Build history of the part. All positions in model axes, mm. A direction names the side the tool comes from. Round coordinates to 2 decimals unless told otherwise and drop trailing zeros. Write each loop counter-clockwise with the first axis right and the second up, starting at its lowest first coordinate (ties: lowest second). Pieces come first, ordered by that corner, then holes. Notation, with made-up numbers: (22, -37) - (46, -37) arc R22 cw to (46, -4) - close; hole circle Ø8 at (-11, -29.5). An arc over 180 degrees is marked (long way). Write each question's results on one line, items separated by ' | '.
from build123d import *

# Parameters (mm, degrees)
SKETCH1_W            = 186
SKETCH1_H            = 166
BOSS_EXTRUDE6_DEPTH  = 3
SKETCH9_W            = 183
SKETCH9_H            = 3
BOSS_EXTRUDE7_DEPTH  = 105
SKETCH8_W            = 3
SKETCH8_H            = 163
BOSS_EXTRUDE8_DEPTH  = 105
SKETCH7_W            = 186
SKETCH7_H            = 3
BOSS_EXTRUDE9_DEPTH  = 105
SKETCH11_W           = 3
SKETCH11_H           = 160
BOSS_EXTRUDE10_DEPTH = 105
SKETCH12_W           = 180
SKETCH12_H           = 3
BOSS_EXTRUDE11_DEPTH = 20
SKETCH13_W           = 45
SKETCH13_H           = 8
CUT_EXTRUDE5_DEPTH   = 3
SKETCH20_W           = 3
SKETCH20_H           = 2
BOSS_EXTRUDE12_DEPTH = 50
SKETCH18_W           = 20
SKETCH18_H           = 20
CUT_EXTRUDE6_DEPTH   = 3
SKETCH22_W           = 3
SKETCH22_H           = 30
BOSS_EXTRUDE13_DEPTH = 6.5
SKETCH23_W           = 3
SKETCH23_H           = 30
BOSS_EXTRUDE15_DEPTH = 20


with BuildPart() as part:
    # Sketch1 → Boss-Extrude6 (new body)
    with BuildSketch(Plane(origin=(0, 0, 0), x_dir=(1, 0, 0), z_dir=(0, 1, 0))):
        with Locations((3.75, -30.125)):
            Rectangle(SKETCH1_W, SKETCH1_H)
    extrude(amount=BOSS_EXTRUDE6_DEPTH)

    # Sketch9 → Boss-Extrude7 (add)
    with BuildSketch(Plane(origin=(0, 3, 0), x_dir=(1, 0, 0), z_dir=(0, 1, 0))):
        with Locations((2.25, -111.625)):
            Rectangle(SKETCH9_W, SKETCH9_H)
    extrude(amount=BOSS_EXTRUDE7_DEPTH)

    # Sketch8 → Boss-Extrude8 (add)
    with BuildSketch(Plane(origin=(0, 3, 0), x_dir=(1, 0, 0), z_dir=(0, 1, 0))):
        with Locations((95.25, -31.625)):
            Rectangle(SKETCH8_W, SKETCH8_H)
    extrude(amount=BOSS_EXTRUDE8_DEPTH)

    # Sketch7 → Boss-Extrude9 (add)
    with BuildSketch(Plane(origin=(0, 3, 0), x_dir=(1, 0, 0), z_dir=(0, 1, 0))):
        with Locations((3.75, 51.375)):
            Rectangle(SKETCH7_W, SKETCH7_H)
    extrude(amount=BOSS_EXTRUDE9_DEPTH)

    # Sketch11 → Boss-Extrude10 (add)
    with BuildSketch(Plane(origin=(0, 3, 0), x_dir=(1, 0, 0), z_dir=(0, 1, 0))):
        with Locations((-87.75, -30.125)):
            Rectangle(SKETCH11_W, SKETCH11_H)
    extrude(amount=BOSS_EXTRUDE10_DEPTH)

    # Sketch12 → Boss-Extrude11 (add)
    with BuildSketch(Plane(origin=(0, 3, 0), x_dir=(1, 0, 0), z_dir=(0, 1, 0))):
        with Locations((3.75, -52.625)):
            Rectangle(SKETCH12_W, SKETCH12_H)
    extrude(amount=BOSS_EXTRUDE11_DEPTH)

    # Sketch13 → Cut-Extrude5 (cut)
    with BuildSketch(Plane(origin=(-86.25, 0, 0), x_dir=(0, 0, -1), z_dir=(1, 0, 0))):
        with Locations((25.375, 7)):
            Rectangle(SKETCH13_W, SKETCH13_H)
    extrude(amount=-CUT_EXTRUDE5_DEPTH, mode=Mode.SUBTRACT)

    # Sketch20 → Boss-Extrude12 (add)
    with BuildSketch(Plane(origin=(0, 3, 0), x_dir=(1, 0, 0), z_dir=(0, 1, 0))):
        with Locations((-81.25, 48.875)):
            Rectangle(SKETCH20_W, SKETCH20_H)
    extrude(amount=BOSS_EXTRUDE12_DEPTH)

    # Sketch18 → Cut-Extrude6 (cut)
    with BuildSketch(Plane.ZY.offset(89.25)):
        with Locations((7.125, 13)):
            Rectangle(SKETCH18_W, SKETCH18_H)
    extrude(amount=-CUT_EXTRUDE6_DEPTH, mode=Mode.SUBTRACT)

    # Sketch22 → Boss-Extrude13 (add)
    with BuildSketch(Plane(origin=(-86.25, 0, 0), x_dir=(0, 0, -1), z_dir=(1, 0, 0))):
        with Locations((1.375, 38)):
            Rectangle(SKETCH22_W, SKETCH22_H)
    extrude(amount=BOSS_EXTRUDE13_DEPTH)

    # Sketch23 → Boss-Extrude15 (add)
    with BuildSketch(Plane(origin=(0, 0, -2.875), x_dir=(-1, 0, 0), z_dir=(0, 0, -1))):
        with Locations((81.25, 38)):
            Rectangle(SKETCH23_W, SKETCH23_H)
    extrude(amount=BOSS_EXTRUDE15_DEPTH)


solid = part.part
(1) Slice it at A-A, the plane y = 87.5. Write the cut outline in (x, z) (3 decimals).
Worked answers:
outline: (-89.25, -52.875) - (96.75, -52.875) - (96.75, 113.125) - (-89.25, 113.125) - close; hole (-86.25, -49.875) - (93.75, -49.875) - (93.75, 110.125) - (-86.25, 110.125) - close
(2) Slice it at B-B, the plane z = 92. Write the cut outline in (x, y).
Worked answers:
outline: (-89.25, 0) - (96.75, 0) - (96.75, 108) - (93.75, 108) - (93.75, 3) - (-86.25, 3) - (-86.25, 108) - (-89.25, 108) - close
(3) Slice it at D-D, the plane z = -32. Write the cut outline in (x, y), and give its area (3 significant figures).
Worked answers:
outline: (-89.25, 0) - (96.75, 0) - (96.75, 108) - (93.75, 108) - (93.75, 3) - (-89.25, 3) - close; (-89.25, 11) - (-86.25, 11) - (-86.25, 108) - (-89.25, 108) - close | area: 1,160 mm2
(4) Drill centre lines: probe 1 along Z at (x, y) = (42, 15) (3 decimals); probe 2 along X at (y, z) = (36, 78); probe 3 along Z at (x, y) = (-60.5, 38) (3 decimals). Where is each one in solid material? Low to high. Write a range as [from, to].
Worked answers:
probe 1: z = [-52.875, -49.875], [51.125, 54.125], [110.125, 113.125] | probe 2: x = [-89.25, -86.25], [93.75, 96.75] | probe 3: z = [-52.875, -49.875], [110.125, 113.125]
(5) Two-plate mould, pull along X, no slides. Class faces 1 (the flat face through (2, 3, 82)), 2 (the flat face through (2, 0, 29)), 3 (the flat face through (-89.25, 53, 31)): released by +X, released by -X, zero draft, split by the parting line, or undercut.
Worked answers:
face 1: undercut | face 2: zero draft | face 3: released by -X
(6) Slice it at C-C, the plane x = 68.5. Write the cut outline in (y, z) (3 decimals).
Worked answers:
outline: (0, -52.875) - (108, -52.875) - (108, -49.875) - (3, -49.875) - (3, 51.125) - (23, 51.125) - (23, 54.125) - (3, 54.125) - (3, 110.125) - (108, 110.125) - (108, 113.125) - (0, 113.125) - close
(7) Flat gauge pin, fed straight in: pin 1 Ø1.6 at (x, z) = (-81.5, -48.5) entering from +Y. Where does the tip first touch, or does it go through?
Worked answers:
pin 1: stops at y = 53
(8) Tool access for faces 4 (the flat face through (3.3, 108, -50.2)), 5 (the flat face through (2, 55, -49.875)), 6 (the flat face through (-84.4, 23, -2.6)): list every direction of +Z, -Z, +X, -X, +Y, -Y with a clear straight run to the whole face (end or side of a thin tool).
Worked answers:
face 4: +Z, -Z, +X, -X, +Y | face 5: +Y | face 6: none
